```python
from build123d import *

# Parameters (mm, degrees)
SKETCH1_R           = 20.6375
BOSS_EXTRUDE1_DEPTH = 76.2
SKETCH2_R           = 3.175
CUT_EXTRUDE1_DEPTH  = 6.35


with BuildPart() as part:
    # Sketch1 → Boss-Extrude1 (new body)
    with BuildSketch(Plane(origin=(0, 0, 0), x_dir=(1, 0, 0), z_dir=(0, 1, 0))):
        with Locations(Location((0, 0, 0), (0, 0, 90))):
            Circle(SKETCH1_R)
    extrude(amount=BOSS_EXTRUDE1_DEPTH)

    # Sketch2 → Cut-Extrude1 (cut)
    with BuildSketch(Plane.XZ):
        with Locations(Location((-10.16, 0, 0), (0, 0, 270))):
            Circle(SKETCH2_R)
        with Locations(Location((10.16, 0, 0), (0, 0, 90))):
            Circle(SKETCH2_R)
    extrude(amount=-CUT_EXTRUDE1_DEPTH, mode=Mode.SUBTRACT)


solid = part.part
```
Input: part model. Units: mm. Frame: model coordinates. A direction names the side the tool comes from. Round coordinates to 2 decimals unless told otherwise and drop trailing zeros. Loops run counter-clockwise (first coordinate to the right, second up) from the corner with the lowest first, then second, coordinate; pieces in that order, holes last. Notation, with made-up numbers: M 40.5,-26 L 94.5,-26 A28 ccw 94.5,-8 Z; hole C 12.5,44.25 d9. An arc over 180 degrees is marked long. Answer in a Markdown table with one row per item. Add a question column.
1. Set-up query: faces 5 (the face through (0, 0, 0)), 6 (the face through (-10, 6.35, 0)). Return all of +Z, -Z, +X, -X, +Y, -Y with unobstructed straight access to the full face (end or side cutting, diameter ignored); none if empty.
2. Section B-B (y = 64). Output: boundary loops of the cut face in (x, z) (1 decimal).
3. Mould query, pull axis X, two halves, no side actions, for faces 1 (the face through (-20.46, 37.57, 2.69)), 2 (the face through (0, 76.2, 0)), 3 (the face through (12.09, 3.13, -2.52)), 4 (the face through (10, 6.35, 0)). Classes: released by +X, released by -X, zero draft, split by the parting line, or undercut.
4. Section C-C (x = -10.16). Output: boundary loops of the cut face in (y, z) (3 decimals).
5. Ray query, probe 1 along X at (y, z) = (3.5, 0) (1 decimal); probe 2 along Z at (x, y) = (10.16, 4.5) (3 decimals); probe 3 along Y at (x, z) = (-13, -0.5). Return the intervals inside material, ascending.
6. Contact query for flat-ended pins moving along their axis: pin 1 (3 mm diameter, centred on x = 10.5, y = 50.5, fed in from -Z); pin 2 (1.9 mm diameter, centred on x = -11, z = 0, fed in from -Y); pin 3 (4 mm diameter, centred on y = 40, z = -5.5, fed in from -X). Output: stop coordinate, or through.
7. Section D-D (x = 4.5). Output: boundary loops of the cut face in (y, z), and give its area (3 significant figures).
Values follow:
| question | item | result |
|---|---|---|
| 1 | face 5 | +Z, -Z, +X, -X, -Y |
| 1 | face 6 | -Y |
| 2 | outline | C 0,0 d41.3 |
| 3 | face 1 | split by the parting line |
| 3 | face 2 | zero draft |
| 3 | face 3 | undercut |
| 3 | face 4 | undercut |
| 4 | outline | M 0,-17.963 L 76.2,-17.963 L 76.2,17.963 L 0,17.963 L 0,3.175 L 6.35,3.175 L 6.35,-3.175 L 0,-3.175 Z |
| 5 | probe 1 | -20.6 to -13.3, -7 to 7, 13.3 to 20.6 |
| 5 | probe 2 | -17.963 to -3.175, 3.175 to 17.963 |
| 5 | probe 3 | 6.35 to 76.2 |
| 6 | pin 1 | z = -18.57 |
| 6 | pin 2 | y = 6.35 |
| 6 | pin 3 | x = -20.34 |
| 7 | outline | M 0,-20.14 L 76.2,-20.14 L 76.2,20.14 L 0,20.14 Z |
| 7 | area | 3,070 mm^2 |
